Geometry: final body of the model. Coordinates: model frame, mm. A direction names the side the tool comes from. Round coordinates to 2 decimals unless told otherwise and drop trailing zeros. Write each loop counter-clockwise with the first axis right and the second up, starting at its lowest first coordinate (ties: lowest second). Pieces come first, ordered by that corner, then holes. Notation, with made-up numbers: (-25.75, 72) -> (-3.75, 72) arc R27 cw to (-3.75, 102) -> close; hole circle Ø5 at (-32, -27.5). An arc over 180 degrees is marked (long way). Use one line per item in the form item = value. Start each with the question number.
1. Cut plane C-C, the plane z = 8.5. Return the cut outline in (x, y).
2. Reachability of faces 1 (the face through (0.6, 6.2, 10.9)), 2 (the face through (5.4, 0.8, 7.9)), 3 (the face through (5, 16, 6.8)), 4 (the face through (5, 14, -8.9)), 5 (the face through (5, 1, -7.9)) from +Z, -Z, +X, -X, +Y, -Y: full face, straight path, thin tool, end or side. Return the list, or none.
3. Draft query along Y for faces 6 (the face through (12.69, 5.94, 10.2)), 7 (the face through (17.4, 13.1, 0.1)), 8 (the face through (5, 3.79, 9)), 9 (the face through (5, 1.6, 0)). Return one class per face: pulls with the +Y half, pulls with the -Y half, needs draft (parallel to the pull), parting line crosses it, or undercut.
4. Cut plane D-D, the plane z = 0. Return the cut outline in (x, y), plus the area to 3 significant figures.
5. Pin query (flat end, axial travel): pin 1 Ø12 at (x, y) = (5.3, 9) entering from -Z; pin 2 Ø1 at (x, z) = (12.5, 9.5) entering from -Y; pin 3 Ø2 at (x, z) = (8.5, 9) entering from -Y; pin 4 Ø8.5 at (x, y) = (5.5, 9) entering from +Z. Return the tip coordinate at first contact, or that it passes through.
6. Cut plane A-A, the plane x = 5.3. State how many separate pieces and enclosed holes the cut face has, plus the area to 3 significant figures.
7. Line query: L1, parallel to Y at x = 5.3, z = 7.35; L2, parallel to Z at x = 6.75, y = 16.5; L3, parallel to Z at x = 3.25, y = 19.25. Output: solid intervals per line, ascending.
```python
from build123d import *

# Parameters (mm, degrees)
EXTRUDE_1_DEPTH     = 24.2
EXTRUDE_2_REACH     = 38.885
SKETCH_2_R          = 8
SKETCH_7_R          = 6.3
CUT_EXTRUDE_5_DEPTH = 2
SKETCH_8_R          = 4.6
CUT_EXTRUDE_6_DEPTH = 37.885363123
EXTRUDE_START       = 1
SKETCH_8_3_R        = 7.8
SKETCH_8_3_R_2      = 4.6
EXTRUDE_3_DEPTH     = 1
CUT_EXTRUDE_7_DEPTH = 22.6


with BuildPart() as part:
    # Sketch 1 → Extrude 1 (new body)
    with BuildSketch(Plane(origin=(0, 0, 0), x_dir=(1, 0, 0), z_dir=(0, 1, 0))):
        with BuildLine():
            Line((0, 7.9), (10.6, 7.9))
            ThreePointArc((10.6, 7.9), (18.5, 0), (10.6, -7.9))
            Line((10.6, -7.9), (0, -7.9))
            ThreePointArc((0, -7.9), (-7.9, 0), (0, 7.9))
        make_face()
    extrude(amount=EXTRUDE_1_DEPTH)

    # Sketch 2 → Extrude 2 (add, up to next)
    with BuildSketch(Plane.XY.offset(12.9), mode=Mode.PRIVATE) as extrude_2_sk1:
        with Locations((5.3, 9)):
            Circle(SKETCH_2_R)
        Polygon((8.307994902, 14.21), (2.292005098, 14.21), (-0.715989805, 9), (2.292005098, 3.79), (8.307994902, 3.79), (11.315989805, 9), align=None, mode=Mode.SUBTRACT)
    extrude_2_tool1 = extrude(extrude_2_sk1.sketch, amount=-EXTRUDE_2_REACH, mode=Mode.PRIVATE) - part.part
    add(extrude_2_tool1.solids().sort_by_distance((-2.473726, 9, 12.9))[0])

    # Sketch 7 → Cut-Extrude 5 (cut)
    with BuildSketch(Plane.XY.offset(12.9)):
        with Locations((5.3, 9)):
            Circle(SKETCH_7_R)
    extrude(amount=-CUT_EXTRUDE_5_DEPTH, mode=Mode.SUBTRACT)

    # Sketch 8 → Cut-Extrude 6 (cut, through all)
    with BuildSketch(Plane(origin=(0, 0, -7.9), x_dir=(-1, 0, 0), z_dir=(0, 0, -1))):
        with Locations((-5.3, 9)):
            Circle(SKETCH_8_R)
    extrude(amount=-CUT_EXTRUDE_6_DEPTH, mode=Mode.SUBTRACT)

    # Sketch 8_3 → Extrude 3 (add)
    with BuildSketch(Plane(origin=(0, 0, -7.9), x_dir=(-1, 0, 0), z_dir=(0, 0, -1)).offset(EXTRUDE_START)):
        with Locations(Location((-5.3, 9, 0), (0, 0, 132.803582426))):
            Circle(SKETCH_8_3_R)
        with Locations((-5.3, 9)):
            Circle(SKETCH_8_3_R_2, mode=Mode.SUBTRACT)
    extrude(amount=-EXTRUDE_3_DEPTH)

    # Sketch 9 → Cut-Extrude 7 (cut)
    with BuildSketch(Plane(origin=(0, 24.2, 0), x_dir=(1, 0, 0), z_dir=(0, 1, 0))):
        with BuildLine():
            Line((10.6, 6.8), (0, 6.8))
            ThreePointArc((0, 6.8), (-6.8, 0), (0, -6.8))
            Line((0, -6.8), (10.6, -6.8))
            ThreePointArc((10.6, -6.8), (17.4, 0), (10.6, 6.8))
        make_face()
    extrude(amount=-CUT_EXTRUDE_7_DEPTH, mode=Mode.SUBTRACT)


solid = part.part
```
Outcome:
q1.outline = circle Ø16 at (5.3, 9); hole (-0.72, 9) -> (2.29, 3.79) -> (8.31, 3.79) -> (11.32, 9) -> (8.31, 14.21) -> (2.29, 14.21) -> close
q2.face_1 = +Z
q2.face_2 = +Z, -Y
q2.face_3 = +Y
q2.face_4 = -Z, +X, -X, +Y, -Y
q2.face_5 = -Z, -Y
q3.face_6 = parting line crosses it
q3.face_7 = needs draft
q3.face_8 = undercut
q3.face_9 = pulls with the +Y half
q4.outline = (-7.9, 0) -> (18.5, 0) -> (18.5, 24.2) -> (17.4, 24.2) -> (17.4, 1.6) -> (-6.8, 1.6) -> (-6.8, 24.2) -> (-7.9, 24.2) -> close
q4.area = 92.0 mm^2
q5.pin_1 = -8.9
q5.pin_2 = 4.63
q5.pin_3 = 1.31
q5.pin_4 = through
q6.separate_pieces = 3
q6.enclosed_holes = 0
q6.area = 84.7 mm^2
q7.L1 = 0 to 4.4, 13.6 to 24.2
q7.L2 = -8.9 to -6.8, 6.8 to 12.9
q7.L3 = -7.9 to -6.8, 6.8 to 7.9
